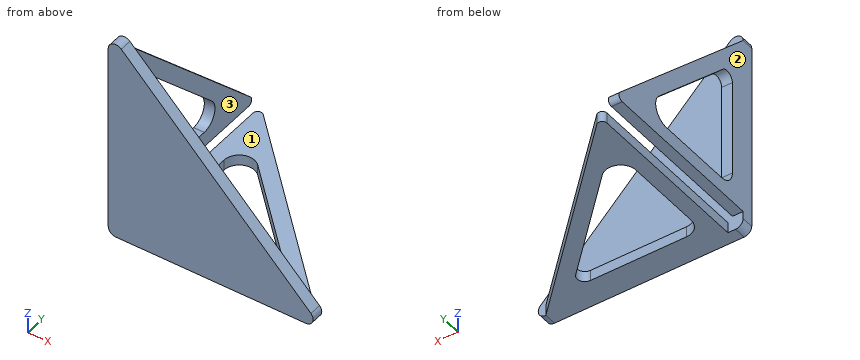
```python
from build123d import *

# Parameters (mm, degrees)
BOSS_EXTRUDE1_DEPTH = 8
EXTRUDE_THIN1_DEPTH = 7
EXTRUDE_THIN2_DEPTH = 7
FILLET1_R           = 10
FILLET2_R           = 5
FILLET3_R           = 3


with BuildPart() as part:
    # Sketch1 → Boss-Extrude1 (new body)
    with BuildSketch(Plane(origin=(0, 0, 0), x_dir=(1, 0, 0), z_dir=(0, 1, 0))):
        with BuildLine():
            Line((8.535533906, -132.885822331), (132.885822331, -8.535533906))
            ThreePointArc((132.885822331, -8.535533906), (133.969686088, -3.086582838), (129.350288425, 0))
            Line((129.350288425, 0), (5, 0))
            ThreePointArc((5, 0), (1.464466094, -1.464466094), (0, -5))
            Line((0, -5), (0, -129.350288425))
            ThreePointArc((0, -129.350288425), (3.086582838, -133.969686088), (8.535533906, -132.885822331))
        make_face()
    extrude(amount=-BOSS_EXTRUDE1_DEPTH)

    # Sketch4 → Extrude-Thin1 (add)
    with BuildSketch(Plane(origin=(0, 0, 0), x_dir=(-1, 0, 0), z_dir=(0, 0, -1))):
        Polygon((-10, 0), (-10, 119.350288425), (-129.350288425, 0), align=None)
        Polygon((-20, 10), (-20, 95.208152802), (-105.208152802, 10), align=None, mode=Mode.SUBTRACT)
    extrude(amount=-EXTRUDE_THIN1_DEPTH)

    # Sketch5 → Extrude-Thin2 (add)
    with BuildSketch(Plane.ZY):
        Polygon((10, 0), (10, 119.350288425), (129.350288425, 0), align=None)
        Polygon((20, 10), (20, 95.208152802), (105.208152802, 10), align=None, mode=Mode.SUBTRACT)
    extrude(amount=-EXTRUDE_THIN2_DEPTH)

    # Fillet1
    fillet1_edges = [part.edges().sort_by_distance(p)[0] for p in [
        (20, 95.208152802, 3.5),
        (20, 10, 3.5),
        (3.5, 95.208152802, 20),
        (3.5, 10, 20),
    ]]
    fillet(fillet1_edges, radius=FILLET1_R)

    # Fillet2
    fillet2_edges = [part.edges().sort_by_distance(p)[0] for p in [
        (105.208152802, 10, 3.5),
        (3.5, 10, 105.208152802),
    ]]
    fillet(fillet2_edges, radius=FILLET2_R)

    # Fillet3
    fillet3_edges = [part.edges().sort_by_distance(p)[0] for p in [
        (10, 119.350288425, 3.5),
        (3.5, 119.350288425, 10),
    ]]
    fillet(fillet3_edges, radius=FILLET3_R)


solid = part.part
```
Input: part model. Units: mm. Frame: model coordinates. Face numbers are marked on the shaded views. A direction names the side the tool comes from. Give positions to 0.01 mm unless a question says otherwise; leave off trailing zeros. Loops run counter-clockwise (first coordinate to the right, second up) from the corner with the lowest first, then second, coordinate; pieces in that order, holes last.
1) Section query C-C on x = 68.5. Return the cut outline in (y, z).
A:
outline: (-8, 0) - (10, 0) - (10, 7) - (0, 7) - (0, 72.92) - (-8, 72.92) - close; (46.71, 0) - (60.85, 0) - (60.85, 7) - (46.71, 7) - close
2) Section query A-A on z = 54.5. Return the cut outline in (x, y), and give its area (3 significant figures).
A:
outline: (0, -8) - (86.92, -8) - (86.92, 0) - (7, 0) - (7, 10) - (0, 10) - close; (0, 60.71) - (7, 60.71) - (7, 74.85) - (0, 74.85) - close
area: 864 mm2
3) Reachability of the marked faces 1, 2 and 3 from +Z, -Z, +X, -X, +Y, -Y: full face, straight path, thin tool, end or side. Return the list, or none.
A:
face 1: +Z, +X, -X, +Y
face 2: +Z, -Z, -X, +Y, -Y
face 3: +Z, -Z, +X, +Y
4) Line query: L1, parallel to X at y = 5, z = 107; L2, parallel to Y at x = 77, z = 55. Output: solid intervals per line, ascending.
A:
L1: x = 0 to 7
L2: y = -8 to 0
5) Contact query for flat-ended pins moving along their axis: pin 1 (10 mm diameter, centred on x = 25, y = 84.5, fed in from +Z); pin 2 (5.5 mm diameter, centred on x = 2.5, y = 55, fed in from +Z); pin 3 (1.5 mm diameter, centred on x = 60, z = 53, fed in from +Y). Output: stop coordinate, or through.
A:
pin 1: stops at z = 7
pin 2: stops at z = 77.1
pin 3: stops at y = 0
6) Section query B-B on y = 106. Return the cut outline in (x, z), and give its area (3 significant figures).
A:
outline: (0, 10) - (7, 10) - (7, 23.35) - (0, 23.35) - close; (10, 0) - (23.35, 0) - (23.35, 7) - (10, 7) - close
area: 187 mm2
7) Section query D-D on y = 37.5. Return the cut outline in (x, z), and give its area (3 significant figures).
A:
outline: (0, 10) - (7, 10) - (7, 20) - (0, 20) - close; (0, 77.71) - (7, 77.71) - (7, 91.85) - (0, 91.85) - close; (10, 0) - (20, 0) - (20, 7) - (10, 7) - close; (77.71, 0) - (91.85, 0) - (91.85, 7) - (77.71, 7) - close
area: 338 mm2
